Answer from the drawing. Dimensions are ordinates in mm from the lowest x, y and z of the part. Round coordinates to 2 decimals unless told otherwise and drop trailing zeros. Write each loop counter-clockwise with the first axis right and the second up, starting at its lowest first coordinate (ties: lowest second). Pieces come first, ordered by that corner, then holes.
1. Straight lines are drawn through the part: probe 1 along Y at (x, z) = (21.5, 1.25); probe 2 along Y at (x, z) = (19.5, 2.3); probe 3 along Y at (x, z) = (44, 0.3). For each, find the intervals that lie inside material, in ascending order.
2. Find section B-B (y = 25). Write down the section's boundary in (x, z), and give its area (3 significant figures).
3. Find section D-D (z = 5.35). Write down the section's boundary in (x, y).
4. Find section C-C (y = 30). Write down the section's boundary in (x, z).
5. Flat-ended cylindrical pins translate along their axes: pin 1 Ø3 at (x, z) = (14, 5) entering from -Y; pin 2 Ø3.5 at (x, y) = (41, 25) entering from +Z; pin 3 Ø1 at (x, z) = (5, 1.5) entering from +Y; pin 4 Ø3 at (x, y) = (8.5, 24) entering from +Z. Find the tip coordinate at first contact, or state that the pin passes through.
6. Find section A-A (x = 25). Write down the section's boundary in (y, z).
7. Determine the mould class of the marked faces 1, 2, 3 and 4 for opening direction X: pulls with the +X half, pulls with the -X half, needs draft (parallel to the pull), parting line crosses it, or undercut.
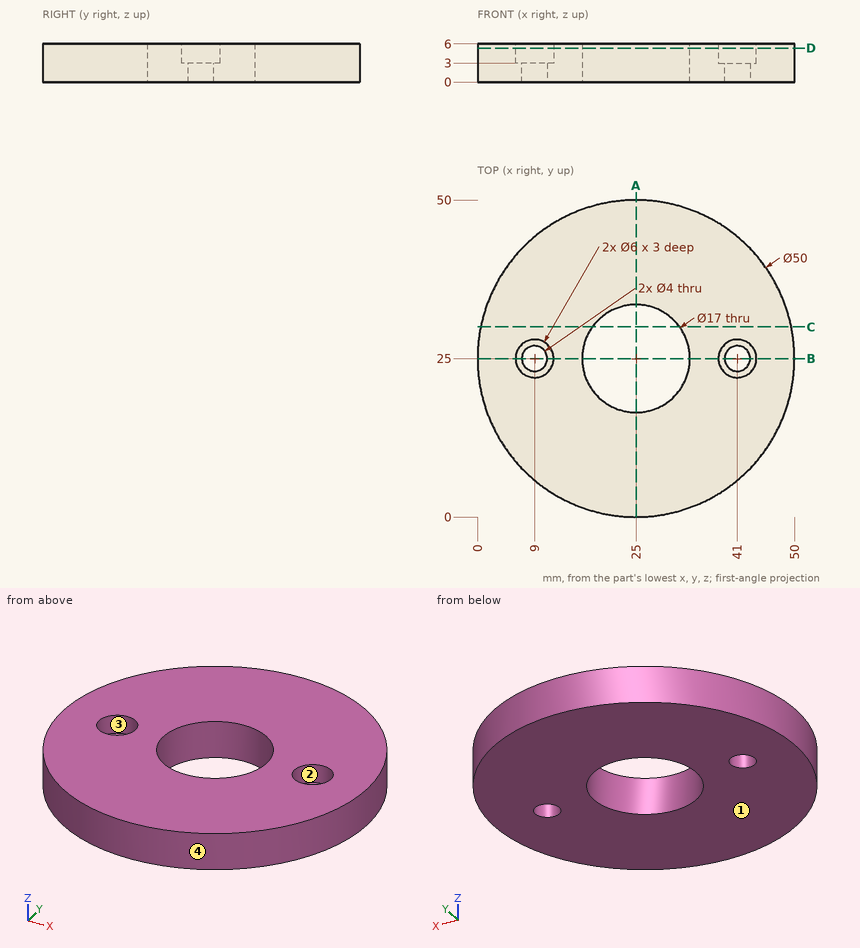
Worked answers:
1. probe 1: y = 0.25 to 17.25, 32.75 to 49.75
1. probe 2: y = 0.61 to 18.52, 31.48 to 49.39
1. probe 3: y = 8.75 to 41.25
2. outline: (0, 0) - (7, 0) - (7, 3) - (6, 3) - (6, 6) - (0, 6) - close; (11, 0) - (16.5, 0) - (16.5, 6) - (12, 6) - (12, 3) - (11, 3) - close; (33.5, 0) - (39, 0) - (39, 3) - (38, 3) - (38, 6) - (33.5, 6) - close; (43, 0) - (50, 0) - (50, 6) - (44, 6) - (44, 3) - (43, 3) - close
2. area: 138 mm2
3. outline: circle Ø50 at (25, 25); hole circle Ø6 at (9, 25); hole circle Ø17 at (25, 25); hole circle Ø6 at (41, 25)
4. outline: (0.51, 0) - (18.13, 0) - (18.13, 6) - (0.51, 6) - close; (31.87, 0) - (49.49, 0) - (49.49, 6) - (31.87, 6) - close
5. pin 1: stops at y = 1.88
5. pin 2: passes through
5. pin 3: stops at y = 40.64
5. pin 4: stops at z = 3
6. outline: (0, 0) - (16.5, 0) - (16.5, 6) - (0, 6) - close; (33.5, 0) - (50, 0) - (50, 6) - (33.5, 6) - close
7. face 1: needs draft
7. face 2: undercut
7. face 3: undercut
7. face 4: parting line crosses it
